Read the model definition and answer for the solid it produces. Units are mm, in the model's axes. A direction names the side the tool comes from. Round coordinates to 2 decimals unless told otherwise and drop trailing zeros. Write each loop counter-clockwise with the first axis right and the second up, starting at its lowest first coordinate (ties: lowest second). Pieces come first, ordered by that corner, then holes. Notation, with made-up numbers: (84, 73) - (95, 73) arc R22 ccw to (95, 92) - close; hole circle Ø4 at (-13.75, 75). An arc over 180 degrees is marked (long way). One line per item, written item: value. Start each with the question number.
(1) Find the intervals of material crossed by L1, parallel to Z at x = -5, y = 5; L2, parallel to X at y = 5.25, z = -4; L3, parallel to Z at x = -3, y = 2, in increasing order.
(2) A cutting plane is placed at A-A, the plane x = -5. Determine the outline of the cut face in (y, z), plus the area to 3 significant figures.
(3) For faces 1 (the face through (-20, 5, 0)), 2 (the face through (-20.9, 9.5, -0.5)), 3 (the face through (-5, 5, -10)), 4 (the face through (-20.9, 0.5, -0.5)), determine the directions among +Z, -Z, +X, -X, +Y, -Y from which every point of the face is accessible in a straight line to the end or side of a thin tool.
(4) A cutting plane is placed at C-C, the plane x = -25. Determine the outline of the cut face in (y, z).
(5) Flat-ended cylindrical pins translate along their axes: pin 1 Ø6 at (x, y) = (-37.5, 7) entering from +Z; pin 2 Ø1.5 at (y, z) = (8, 0.5) entering from +X. Find the tip coordinate at first contact, or state that the pin passes through.
(6) A cutting plane is placed at B-B, the plane y = 3.25. Determine the outline of the cut face in (x, z), plus the area to 3 significant figures.
Autodesk Fusion 360 part; units mm, degrees
sketch "Sketch3" plane through (0, 0, 0) normal (0, 1, 0) x (1, 0, 0)
  line L0 (0, 0) -> (-40, 0)
  line L1 (-40, 0) -> (-49.3969, -3.4202)
  line L2 (-40, 0) -> (-30, 0) construction
  line L3 (-49.3969, -3.4202) -> (-49.3969, -0.4202)
  line L4 (-49.3969, -0.4202) -> (-40.7346, 4.5763)
  line L5 (0, 0) -> (0, 10)
  line L6 (0, 10) -> (-10, 10)
  line L7 (-10, 10) -> (-40.7346, 4.5763)
  dimension "d3" = 40
  dimension "d4" = 160
  dimension "d5" = 10
  dimension "d6" = 3
  dimension "d7" = 10
  dimension "d8" = 10
  dimension "d9" = 10
extrude "Extrude1" add sketch "Sketch3" along normal blind 10
sketch "Sketch4" plane through (0, 10, 0) normal (0, 1, 0) x (-1, 0, 0)
  line L0 (0, 0) -> (0, -10)
  line L1 (0, -10) -> (10, -10)
  line L2 (10, -10) -> (40.7346, -4.5763)
  line L3 (40.7346, -4.5763) -> (49.3969, 0.4202)
  line L4 (49.3969, 0.4202) -> (49.3969, 3.4202)
  line L5 (49.3969, 3.4202) -> (40, 0)
  line L6 (40, 0) -> (0, 0)
  line L7 (0, 0) -> (10, 0)
  line L8 (0, -5) -> (5, -4.9937)
  circle A0 centre (5, -4.9937) radius 3.2
  dimension "d12" = 10
  dimension "d26" = 5
  dimension "d27" = 6.4
sketch "Sketch5" plane through (0, 0, 0) normal (0, -1, 0) x (1, 0, 0)
  line L0 (0, -10) -> (0, 0)
  line L1 (0, 0) -> (-40, 0)
  line L2 (-40, 0) -> (-49.3969, 3.4202)
  line L3 (-49.3969, 3.4202) -> (-49.3969, 0.4202)
  line L4 (-49.3969, 0.4202) -> (-40.7346, -4.5763)
  line L5 (-40.7346, -4.5763) -> (-10, -10)
  line L6 (-10, -10) -> (0, -10)
  line L7 (0, 0) -> (-10, 0)
  dimension "d13" = 10
extrude "Extrude2" cut sketch "Sketch4" against normal blind 21 contours A0
chamfer "Chamfer1" distance 1 angle 45 8 edges at (0, 5, -10) (0, 5, 0) (-5, 10, -10) (0, 10, -5) (-20, 10, 0) (-20, 0, 0) (0, 0, -5) (-5, 0, -10)
chamfer "Chamfer2" distance 1 angle 45 1 edges at (-43.3247, 10, 1.2101)
chamfer "Chamfer3" distance 1 angle 45 1 edges at (-45.0658, 10, -2.078)
chamfer "Chamfer4" distance 1 angle 45 1 edges at (-28.2007, 0, -6.7881)
chamfer "Chamfer5" distance 1 angle 45 1 edges at (-26.7588, 10, -7.0426)
chamfer "Chamfer6" distance 1 angle 45 1 edges at (-40.7346, 5, -4.5763)
chamfer "Chamfer7" distance 1 angle 45 1 edges at (-49.3969, 4.5, 0.4202)
chamfer "Chamfer8" distance 1 angle 45 1 edges at (-45.9009, 0, -1.5963)
chamfer "Chamfer9" distance 1 angle 45 1 edges at (-43.3247, 0, 1.2101)
chamfer "Chamfer10" distance 1 angle 45 1 edges at (-49.3969, 5, 3.4202)
chamfer "Chamfer11" distance 0.5 angle 70 2 edges at (-2.0165, 0, -6.1508) (-2.0165, 10, -3.8365) measured on face at (-19.4177, 0, -4.8389) measured on face at (-19.4177, 10, -4.8389)
equation "d14 = ElephantFIT"
equation "ElephantFIT = 1 mm"
equation "d16 = StyleFIT"
equation "d17 = StyleFIT"
equation "d18 = StyleFIT"
equation "d19 = StyleFIT"
equation "d20 = StyleFIT"
equation "d21 = StyleFIT"
equation "d22 = StyleFIT"
equation "d23 = StyleFIT"
equation "d24 = StyleFIT"
equation "StyleFIT = 1 mm"
equation "d26 = HolePosX"
equation "d27 = HoleSize"
equation "HoleSize = 6.4 mm"
equation "HolePosX = 5 mm"
equation "d32 = HoleFIT"
equation "d33 = HoleAngle"
equation "HoleFIT = 0.5 mm"
equation "HoleAngle = 70 deg"
Here are the results:
1. L1: -10 to -8.19, -1.79 to 0
1. L2: -41.73 to -8.04, -1.96 to 0
1. L3: -10 to -7.49, -2.5 to 0
2. outline: (0, -9) - (1, -10) - (9, -10) - (10, -9) - (10, -8.69) - (8.63, -8.19) - (1.37, -8.19) - (0, -8.69) - close; (0, -1.29) - (1.37, -1.79) - (8.63, -1.79) - (10, -1.29) - (10, -1) - (9, 0) - (1, 0) - (0, -1) - close
2. area: 32.6 mm²
3. face 1: +Z, +X, +Y, -Y
3. face 2: +Z, +X, +Y
3. face 3: -Z, +X, -X, +Y, -Y
3. face 4: +Z, +X, -Y
4. outline: (0, -6.34) - (1, -7.35) - (9, -7.35) - (10, -6.34) - (10, -1) - (9, 0) - (1, 0) - (0, -1) - close
5. pin 1: z = 0.18
5. pin 2: x = -0.75
6. outline: (-49.4, 1.42) - (-48.53, -0.08) - (-41.6, -4.08) - (-39.75, -4.75) - (-10, -10) - (-1, -10) - (0, -9) - (0, -1) - (-1, 0) - (-40, 0) - (-48.46, 3.08) - (-49.4, 2.42) - close; hole circle Ø6.4 at (-5, -4.99)
6. area: 324 mm²
